Geometry: see drawing. Coordinates: mm, zero at the bounding-box minimum. A direction names the side the tool comes from. Coordinates: 2 decimals unless noted, no trailing zeros. Order: outer loops, then holes, each group sorted by start corner. A loop starts at its lowest first (then second) coordinate and runs counter-clockwise, first axis right, second up. Notation, with made-up numbers: (78.25, 41) -> (113.25, 41) arc R17 cw to (113.25, 59) -> close; hole circle Ø11 at (74.5, -10.5). An arc over 180 degrees is marked (long way). Use one line per item in the form item = value.
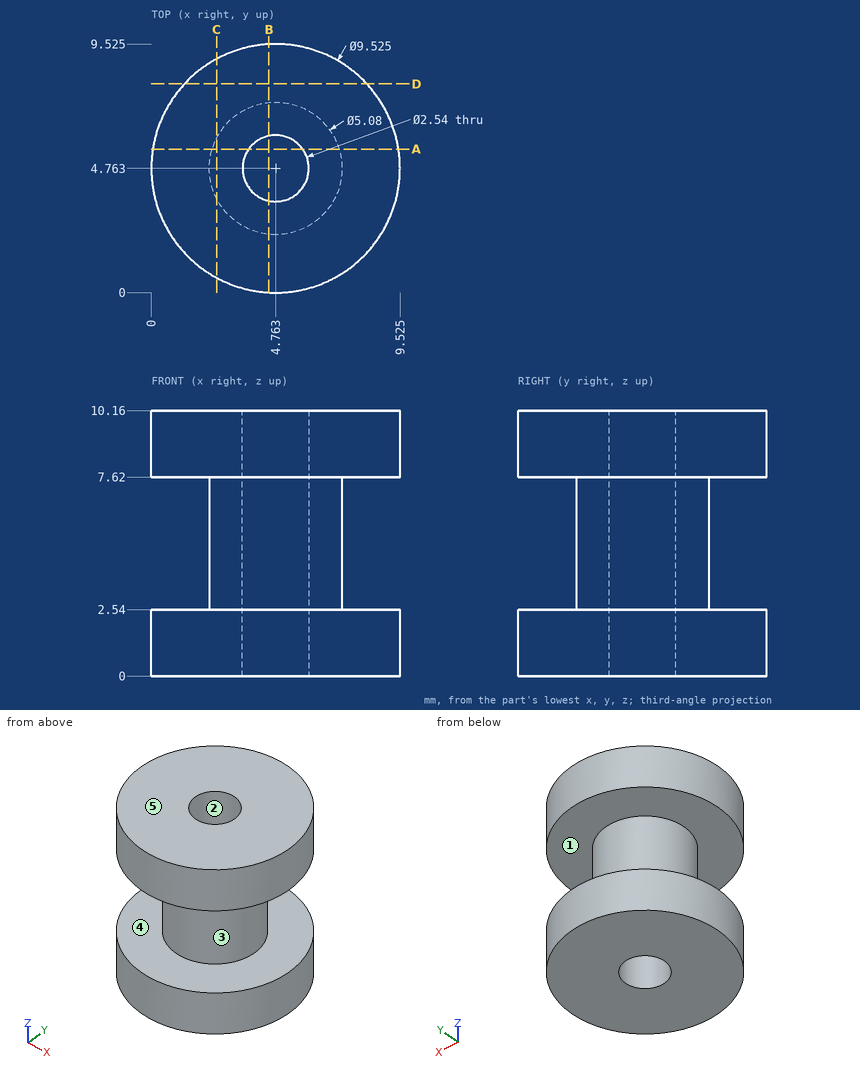
1) Pull-direction query (X, two-part tool) for the marked faces 1, 2 and 3; classes: released by +X, released by -X, zero draft, split by the parting line, or undercut.
Results found:
face_1 = zero draft
face_2 = undercut
face_3 = split by the parting line
2) Access query for the marked faces 4 and 5. Directions: +Z, -Z, +X, -X, +Y, -Y. A direction counts if a zero-diameter tool reaches every point of the face in a straight line with its end or side. Return the directions, or none.
Results found:
face_4 = none
face_5 = +Z, +X, -X, +Y, -Y
3) Section D-D, the plane y = 8. Output: boundary loops of the cut face in (x, z) (1 decimal).
Results found:
outline = (1.3, 0) -> (8.3, 0) -> (8.3, 2.5) -> (1.3, 2.5) -> close; (1.3, 7.6) -> (8.3, 7.6) -> (8.3, 10.2) -> (1.3, 10.2) -> close
4) Contact query for a flat-ended pin moving along its axis: P1, Ø5, axis at y = 5.5, z = 2, coming from the +X side (1 decimal). Output: stop coordinate, or through.
Results found:
P1 = 9.5
5) Section B-B, the plane x = 4.5. Output: boundary loops of the cut face in (y, z) (1 decimal).
Results found:
outline = (0, 0) -> (3.5, 0) -> (3.5, 10.2) -> (0, 10.2) -> (0, 7.6) -> (2.2, 7.6) -> (2.2, 2.5) -> (0, 2.5) -> close; (6, 0) -> (9.5, 0) -> (9.5, 2.5) -> (7.3, 2.5) -> (7.3, 7.6) -> (9.5, 7.6) -> (9.5, 10.2) -> (6, 10.2) -> close
6) Material intervals for probe 1 along Z at (x, y) = (7.25, 8.5); probe 2 along Y at (x, z) = (4.75, 8.5) (1 decimal); probe 3 along X at (y, z) = (4.75, 4.5), sorted ascending. Write a range as from..to.
Results found:
probe_1 = 0..2.54, 7.62..10.16
probe_2 = 0..3.5, 6..9.5
probe_3 = 2.22..3.49, 6.03..7.3
7) Section A-A, the plane y = 5.5. Output: boundary loops of the cut face in (x, z).
Results found:
outline = (0.06, 0) -> (3.73, 0) -> (3.73, 10.16) -> (0.06, 10.16) -> (0.06, 7.62) -> (2.33, 7.62) -> (2.33, 2.54) -> (0.06, 2.54) -> close; (5.8, 0) -> (9.47, 0) -> (9.47, 2.54) -> (7.19, 2.54) -> (7.19, 7.62) -> (9.47, 7.62) -> (9.47, 10.16) -> (5.8, 10.16) -> close
8) Section C-C, the plane x = 2.5. Output: boundary loops of the cut face in (y, z).
Results found:
outline = (0.57, 0) -> (8.95, 0) -> (8.95, 2.54) -> (5.92, 2.54) -> (5.92, 7.62) -> (8.95, 7.62) -> (8.95, 10.16) -> (0.57, 10.16) -> (0.57, 7.62) -> (3.61, 7.62) -> (3.61, 2.54) -> (0.57, 2.54) -> close
